Input: part model. Units: mm. Frame: model coordinates. Face numbers are marked on the shaded views. Give positions to 0.01 mm unless a question says otherwise; leave off trailing zeros. Write each loop counter-clockwise with the first axis right and the second up, starting at its lowest first coordinate (ties: lowest second). Pieces come first, ordered by that corner, then holes. Notation, with made-up numbers: (-23.5, 23.5) - (27.5, 23.5) arc R14 ccw to (27.5, 41.5) - close; hole circle Ø9 at (-10.75, 56.5). An arc over 180 degrees is marked (long way). Answer as CSV lines item,"result". Start each with the question number.
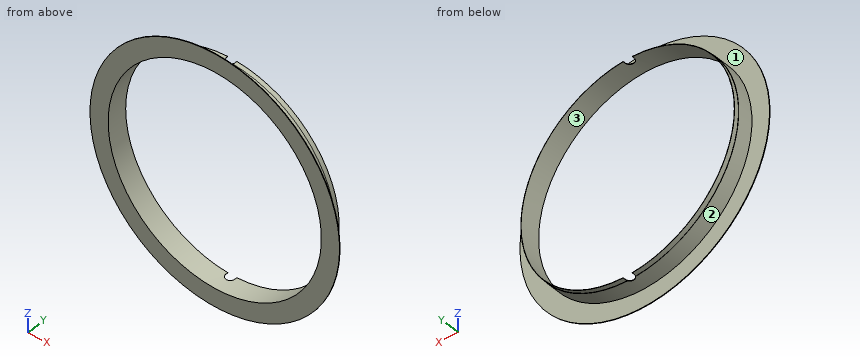
Autodesk Inventor part; units mm, degrees
ref_plane "Work Plane1" through (0, 0.3969, 174.625) normal (0, 0, 1) x (1, 0, 0)
ref_plane "YZ Plane" through (0, 0, 0) normal (1, 0, 0) x (0, 1, 0)
ref_plane "XZ Plane" through (0, 0, 0) normal (0, 1, 0) x (-1, 0, 0)
sketch "Sketch1" plane through (0, 0, 0) normal (1, 0, 0) x (0, 1, 0)
  line L0 (0, 0) -> (1.9826, 0)
  line L1 (0, 149.225) -> (25.4, 149.225)
  line L2 (0, 149.225) -> (0, 174.625)
  line L3 (0, 174.625) -> (0.7937, 174.625)
  line L4 (0.7937, 174.625) -> (0.7937, 150.0187)
  line L5 (0.7937, 150.0187) -> (22.225, 150.0187)
  line L6 (25.4, 149.6219) -> (25.4, 149.225)
  line L7 (25.4, 149.225) -> (28.575, 149.225)
  line L8 (28.575, 149.225) -> (28.575, 149.6219)
  line L9 (28.575, 149.6219) -> (22.225, 149.6219)
  line L10 (22.225, 149.6219) -> (22.225, 150.0187)
  point P0 (0.3969, 174.625)
  dimension "d0" = 25.4
  dimension "d1" = 149.225
  dimension "d2" = 25.4
  dimension "d3" = 0.7937
  dimension "d4" = 24.6062
  dimension "d5" = 3.175
  dimension "d6" = 6.35
revolve "Revolution1" add sketch "Sketch1" angle 360 about axis through (0, 0, 0) along (0, 1, 0)
ref_plane "Work Plane1" through (0, 0.3969, 174.625) normal (0, 0, 1) x (1, 0, 0)
sketch "Sketch2" plane through (0, 0.3969, 174.625) normal (0, 0, 1) x (1, 0, 0)
  line L0 (149.6219, 28.1781) -> (-149.6219, 28.1781)
  arc A0 (-6.35, 25.0031) -> (6.35, 25.0031) centre (0, 25.0031) ccw
  line L1 (-6.35, 25.0031) -> (-6.35, 28.1781)
  line L2 (6.35, 25.0031) -> (6.35, 28.1781)
  line L3 (149.225, 28.1781) -> (-149.225, 28.1781)
  line L4 (-6.35, 28.1781) -> (6.35, 28.1781)
  point P0 (0, -0.3969)
  dimension "d8" = 3.175
  dimension "d9" = 0
  dimension "d10" = 12.7
extrude "Extrusion1" cut sketch "Sketch2" against normal through all
properties part number "Layer2_Bottom"
1) Contact query for flat-ended pins moving along their axis: P1, Ø3, axis at x = -96, y = 8, coming from the +Z side; P2, Ø4, axis at y = 13, z = 35.5, coming from the +X side; P3, Ø1, axis at x = -70, z = 133, coming from the +Y side (3 decimals). Output: stop coordinate, or through.
2) Pull-direction query (X, two-part tool) for the marked faces 1, 2 and 3; classes: +X half, -X half, draft (parallel to the pull), parting line (faces both ways), or undercut.
3) Cut plane A-A on x = 0. Output: boundary loops of the cut face in (y, z) (3 decimals), and give its area (3 significant figures).
4) Material intervals for line 1 (Z direction, x = 0, y = 9.5) (3 decimals); line 2 (X direction, y = 21.75, z = 5), sorted ascending. Write a range as from..to.
5) Cut plane B-B on z = 0. Output: boundary loops of the cut face in (x, y) (3 decimals).
6) Cut plane C-C on y = 10.25. Output: boundary loops of the cut face in (x, z) (3 decimals).
7) Cut plane D-D on z = -67. Output: boundary loops of the cut face in (x, y) (3 decimals).
Numbers:
1,P1,"stops at z = 116.51"
1,P2,"stops at x = 146.23"
1,P3,"stops at y = 22.225"
2,face 1,"draft"
2,face 2,"parting line"
2,face 3,"undercut"
3,outline,"(0, -174.625) - (0.794, -174.625) - (0.794, -150.019) - (19.05, -150.019) - (19.05, -149.225) - (0, -149.225) - close; (0, 149.225) - (19.05, 149.225) - (19.05, 150.019) - (0.794, 150.019) - (0.794, 174.625) - (0, 174.625) - close"
3,area,"69.3 mm²"
4,line 1,"z = -150.019..-149.225, 149.225..150.019"
4,line 2,"x = -149.94..-149.14, 149.14..149.94"
5,outline,"(-174.625, 0) - (-149.225, 0) - (-149.225, 28.575) - (-149.622, 28.575) - (-149.622, 22.225) - (-150.019, 22.225) - (-150.019, 0.794) - (-174.625, 0.794) - close; (149.225, 0) - (174.625, 0) - (174.625, 0.794) - (150.019, 0.794) - (150.019, 22.225) - (149.622, 22.225) - (149.622, 28.575) - (149.225, 28.575) - close"
6,outline,"circle Ø300.037 at (0, 0); hole circle Ø298.45 at (0, 0)"
7,outline,"(-161.26, 0) - (-133.338, 0) - (-133.338, 28.575) - (-133.782, 28.575) - (-133.782, 22.225) - (-134.226, 22.225) - (-134.226, 0.794) - (-161.26, 0.794) - close; (133.338, 0) - (161.26, 0) - (161.26, 0.794) - (134.226, 0.794) - (134.226, 22.225) - (133.782, 22.225) - (133.782, 28.575) - (133.338, 28.575) - close"
